from build123d import *

# Parameters (mm, degrees)
SKETCH_1_R          = 1
SKETCH_1_R_2        = 1.5
EXTRUDE_1_DEPTH     = 6
SKETCH_3_W          = 15
SKETCH_3_H          = 4
CUT_EXTRUDE_1_DEPTH = 10


with BuildPart() as part:
    # Эскиз1 → Бобышка-Вытянуть1 (new body)
    with BuildSketch(Plane.XY):
        with BuildLine():
            Line((0, 0), (0, 32))
            Line((0, 32), (1.872137409, 32))
            ThreePointArc((1.872137409, 32), (3.069970858, 29.210301659), (5, 26.866755347))
            Line((5, 26.866755347), (5, 0))
            Line((5, 0), (19.5, 0))
            Line((19.5, 0), (19.5, 26.866755347))
            ThreePointArc((19.5, 26.866755347), (22.14801609, 30.609753984), (22.995479479, 35.115731548))
            Line((22.995479479, 35.115731548), (22.995479479, 39.473981947))
            ThreePointArc((22.995479479, 39.473981947), (43.022434445, 48.648827827), (50.6, 27.964601411))
            ThreePointArc((50.6, 27.964601411), (49.778888952, 25.750204045), (49.5, 23.404996165))
            Line((49.5, 23.404996165), (49.5, -4))
            Line((49.5, -4), (0, -4))
            Line((0, -4), (0, 0))
        make_face()
        with Locations((2, 27)):
            Circle(SKETCH_1_R, mode=Mode.SUBTRACT)
        with Locations(Location((22.5, 27, 0), (0, 0, 180))):
            Circle(SKETCH_1_R, mode=Mode.SUBTRACT)
        with Locations((22.5, 6)):
            Circle(SKETCH_1_R, mode=Mode.SUBTRACT)
        with Locations(Location((2, 6, 0), (0, 0, 180))):
            Circle(SKETCH_1_R, mode=Mode.SUBTRACT)
        with Locations((37.25, 34.80400928)):
            Circle(SKETCH_1_R_2, mode=Mode.SUBTRACT)
    extrude(amount=EXTRUDE_1_DEPTH)

    # Эскиз3 → Вырез-Вытянуть1 (cut)
    with BuildSketch(Plane.XY.offset(6)):
        with Locations((34.5, -2)):
            Rectangle(SKETCH_3_W, SKETCH_3_H)
    extrude(amount=-CUT_EXTRUDE_1_DEPTH, mode=Mode.SUBTRACT)


solid = part.part
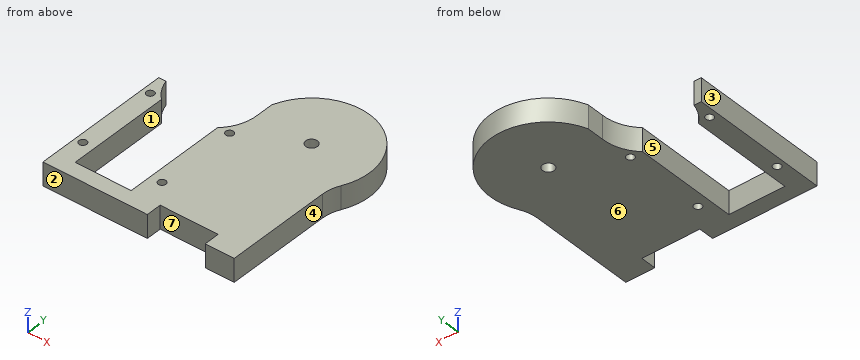
Geometry: final body of the model. Coordinates: model frame, mm. Face numbers are marked on the shaded views. A direction names the side the tool comes from. Give positions to 0.01 mm unless a question says otherwise; leave off trailing zeros. Write each loop counter-clockwise with the first axis right and the second up, starting at its lowest first coordinate (ties: lowest second). Pieces come first, ordered by that corner, then holes.
(1) First-contact query: P1, Ø1.8, axis at y = 13, z = 4.5, coming from the +X side; P2, Ø1.3, axis at y = 37, z = 3.5, coming from the -X side; P3, Ø3, axis at x = 12, z = 3.5, coming from the +Y side. Flat tips, straight axial feed; report the tip coordinate or a pass-through.
(2) Cut plane B-B, the plane y = 16.5. Return loops of the section in (x, z), then the cut area to 3 significant figures.
(3) Ray query, line 1 (X direction, y = 21.5, z = 1.7); line 2 (Y direction, x = 37.25, z = 2.2); line 3 (Y direction, x = 6.5, z = 5.2). Return the intervals inside material, ascending.
(4) Mould query, pull axis X, two halves, no side actions, for the marked faces 1, 2, 3 and 4. Classes: released by +X, released by -X, zero draft, split by the parting line, or undercut.
(5) Cut plane A-A, the plane y = 6. Return loops of the section in (x, z), then the cut area to 3 significant figures.
(6) Cut plane C-C, the plane z = 1.55. Return loops of the section in (x, y) (3 decimals).
(7) Cut plane D-D, the plane x = 11. Return loops of the section in (y, z), then the cut area to 3 significant figures.
(8) Access query for the marked faces 5, 6 and 7. Directions: +Z, -Z, +X, -X, +Y, -Y. A direction counts if a zero-diameter tool reaches every point of the face in a straight line with its end or side. Return the directions, or none.
Values follow:
1. P1: stops at x = 49.5
1. P2: stops at x = 23
1. P3: stops at y = 0
2. outline: (0, 0) - (5, 0) - (5, 6) - (0, 6) - close; (19.5, 0) - (49.5, 0) - (49.5, 6) - (19.5, 6) - close
2. area: 210 mm2
3. line 1: x = 0 to 5, 19.5 to 49.5
3. line 2: y = 0 to 33.3, 36.3 to 49.8
3. line 3: y = -4 to 0
4. face 1: undercut
4. face 2: zero draft
4. face 3: released by -X
4. face 4: released by +X
5. outline: (0, 0) - (1, 0) - (1, 6) - (0, 6) - close; (3, 0) - (5, 0) - (5, 6) - (3, 6) - close; (19.5, 0) - (21.5, 0) - (21.5, 6) - (19.5, 6) - close; (23.5, 0) - (49.5, 0) - (49.5, 6) - (23.5, 6) - close
5. area: 186 mm2
6. outline: (0, -4) - (27, -4) - (27, 0) - (42, 0) - (42, -4) - (49.5, -4) - (49.5, 23.405) arc R10 cw to (50.6, 27.965) arc R15 ccw (long way) to (22.995, 39.474) - (22.995, 35.116) arc R10.75 cw to (19.5, 26.867) - (19.5, 0) - (5, 0) - (5, 26.867) arc R10.75 cw to (1.872, 32) - (0, 32) - close; hole circle Ø2 at (2, 6); hole circle Ø2 at (2, 27); hole circle Ø2 at (22.5, 6); hole circle Ø2 at (22.5, 27); hole circle Ø3 at (37.25, 34.804)
7. outline: (-4, 0) - (0, 0) - (0, 6) - (-4, 6) - close
7. area: 24.0 mm2
8. face 5: +Z, -Z, +Y
8. face 6: -Z, +X, -X, +Y, -Y
8. face 7: +Z, -Z, -Y
